Here's the drawing with two shaded views (mm, measured from the low corner). I have some questions. Round coordinates to 2 decimals unless told otherwise and drop trailing zeros. Loops run counter-clockwise (first coordinate to the right, second up) from the corner with the lowest first, then second, coordinate; pieces in that order, holes last.
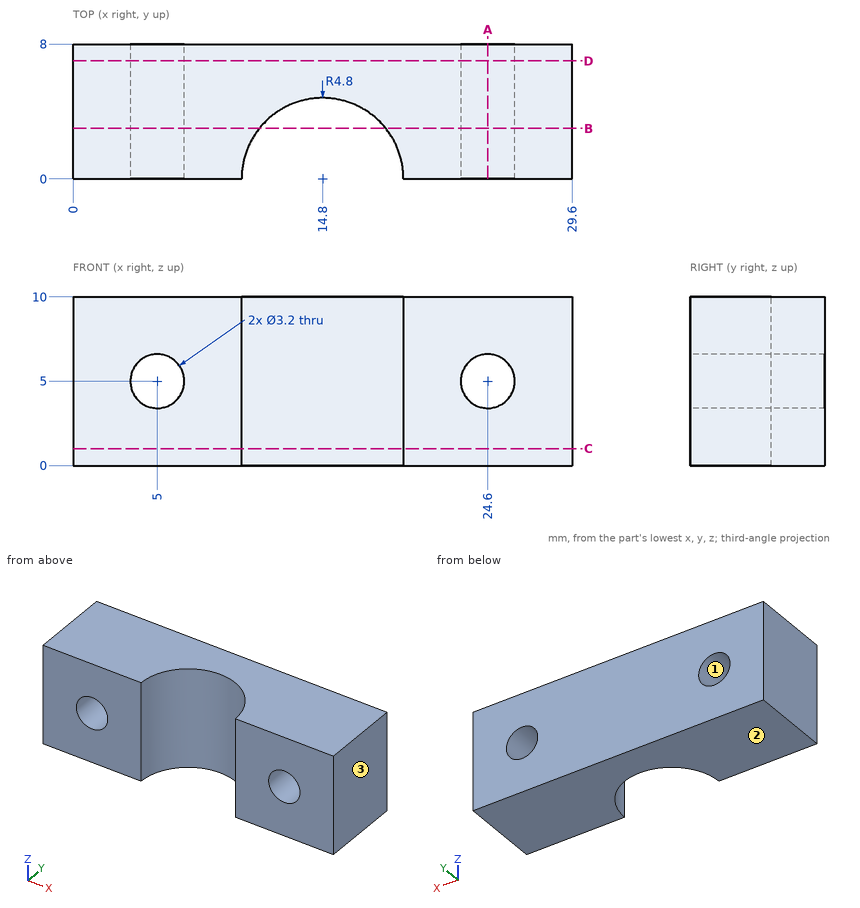
Item 1: If I drill on line 1 along Z through (x, y) = (5, 6); line 2 along X through (y, z) = (1, 7.5); line 3 along Z through (x, y) = (25.5, 3), over which ranges is the centre line in solid material (lowest first)?
Results list:
line 1: z = 0 to 3.4, 6.6 to 10
line 2: x = 0 to 10.11, 19.49 to 29.6
line 3: z = 0 to 3.68, 6.32 to 10
Item 2: If we section it at C-C, the plane z = 1: Please give me the cut outline in (x, y).
Results list:
outline: (0, 0) - (10, 0) arc R4.8 cw to (19.6, 0) - (29.6, 0) - (29.6, 8) - (0, 8) - close
Item 3: If we section it at A-A, the plane x = 24.6: Please give me the cut outline in (y, z), then the cut area to 3 significant figures.
Results list:
outline: (0, 0) - (8, 0) - (8, 3.4) - (0, 3.4) - close; (0, 6.6) - (8, 6.6) - (8, 10) - (0, 10) - close
area: 54.4 mm2
Item 4: If we section it at D-D, the plane y = 7: Please give me the cut outline in (x, z), then the cut area to 3 significant figures.
Results list:
outline: (0, 0) - (29.6, 0) - (29.6, 10) - (0, 10) - close; hole circle Ø3.2 at (5, 5); hole circle Ø3.2 at (24.6, 5)
area: 280 mm2
Item 5: Will these pins go through, and if not, where does the flat tip stop? pin 1 (2.5 mm diameter, centred on x = 24.6, z = 5, fed in from +Y); pin 2 (1 mm diameter, centred on x = 19.5, z = 7, fed in from -Y).
Results list:
pin 1: passes through
pin 2: stops at y = 0
Item 6: We'd pull the mould along Z, two halves only. Please class the marked faces 1, 2 and 3: released by +Z, released by -Z, zero draft, split by the parting line, or undercut.
Results list:
face 1: undercut
face 2: released by -Z
face 3: zero draft
Item 7: If we section it at B-B, the plane y = 3: Please give me the cut outline in (x, z).
Results list:
outline: (0, 0) - (11.05, 0) - (11.05, 10) - (0, 10) - close; (18.55, 0) - (29.6, 0) - (29.6, 10) - (18.55, 10) - close; hole circle Ø3.2 at (5, 5); hole circle Ø3.2 at (24.6, 5)
